The listing builds one solid part. Answer for the finished solid, in the listing's coordinates (mm). Coordinates: 2 decimals unless noted, no trailing zeros. Loops run counter-clockwise (first coordinate to the right, second up) from the corner with the lowest first, then second, coordinate; pieces in that order, holes last. Notation, with made-up numbers: (-18.75, -3) - (16.25, -3) arc R12 ccw to (16.25, 5) - close; hole circle Ø3 at (-31.5, -35). An arc over 180 degrees is marked (long way). Put each result on its own line as item: value.
Autodesk Inventor part; units mm, degrees
ref_plane "YZ Plane" through (0, 0, 0) normal (1, 0, 0) x (0, 1, 0)
ref_plane "XZ Plane" through (0, 0, 0) normal (0, 1, 0) x (-1, 0, 0)
ref_plane "XY Plane" through (0, 0, 0) normal (0, 0, 1) x (1, 0, 0)
sketch "Sketch1" plane through (0, 0, 0) normal (0, 1, 0) x (-1, 0, 0)
  line L0 (25, 100) -> (-25, 100)
  line L1 (-25, 100) -> (-25, -100)
  line L2 (-25, -100) -> (25, -100)
  line L3 (25, -100) -> (25, 100)
  line L4 (25, 100) -> (-25, -100) construction
  line L5 (-25, 100) -> (25, -100) construction
  point P0 (0, 0)
  dimension "d0" = 50
  dimension "d1" = 200
extrude "Extrusion1" add sketch "Sketch1" along normal blind 62
sketch "Sketch2" plane through (-25, 0, 100) normal (0, 0, 1) x (1, 0, 0)
  line L0 (50, 62) -> (0, 62)
  line L1 (50, 62) -> (90, 62)
  line L2 (90, 62) -> (90, 42)
  line L3 (90, 42) -> (53.2289, 0)
  line L4 (53.2289, 0) -> (50, 0)
  line L5 (50, 62) -> (50, 0)
  point P0 (25, 0)
  dimension "d4" = 40
  dimension "d5" = 20
  dimension "d6" = 90
extrude "Extrusion2" add sketch "Sketch2" against normal up to surface (200 mm away)
sketch "Sketch3" plane through (0, 62, 0) normal (0, 1, 0) x (1, 0, 0)
  line L0 (-25, 100) -> (-25, -100)
  line L1 (-25, -100) -> (-25, 100)
  line L2 (-25, 100) -> (-25, 80)
  line L3 (-25, 80) -> (-76.9615, 50)
  line L4 (-25, -100) -> (-25, -80)
  line L5 (-25, -80) -> (-76.9615, -50)
  line L6 (-76.9615, -50) -> (-76.9615, 50)
  circle A0 centre (-76.9615, 0) radius 49.9974
  circle A1 centre (-126.9564, -0.5064) radius 49.9974
  line L7 (-76.9615, -50) -> (-126.45, -50.5013)
  line L8 (-127.4628, 49.4885) -> (-76.9615, 50)
  point P0 (0, 0)
  point P1 (-76.9615, 49.9974)
  point P2 (-77.4679, 49.9949)
  point P3 (-76.9615, -1.0128)
  dimension "d9" = 20
  dimension "d10" = 60
  dimension "d11" = 120
  dimension "d12" = 20
  dimension "d13" = 60
  dimension "d14" = 120
extrude "Extrusion3" add sketch "Sketch3" against normal blind 62
sketch "Sketch4" plane through (0, 62, 0) normal (0, 1, 0) x (1, 0, 0)
  line L0 (-25, -100) -> (28.2289, -100)
  line L1 (-25, 100) -> (-25, 80)
  line L2 (-25, -100) -> (-25, 100)
  line L3 (-25, 100) -> (29.4775, 197.567)
  line L4 (29.4775, 197.567) -> (135.6867, 127.811)
  line L5 (135.6867, 127.811) -> (135.6867, -104.409)
  line L6 (135.6867, -104.409) -> (110.0345, -245.7212)
  line L7 (110.0345, -245.7212) -> (-5.1754, -156.6135)
  line L8 (-5.1754, -156.6135) -> (-25, -100)
  line L9 (-76.9615, -50) -> (-76.9615, 49.9974)
  line L10 (-76.9615, 49.9974) -> (-143.8651, 145.0549)
  line L11 (-143.8651, 145.0549) -> (-248.9816, -0.0013)
  line L12 (-248.9816, -0.0013) -> (-240.1494, -166.1828)
  line L13 (-240.1494, -166.1828) -> (-110.4133, -169.4443)
  line L14 (-110.4133, -169.4443) -> (-76.9615, -50)
  point P0 (0, 0)
extrude "Extrusion4" cut sketch "Sketch4" against normal blind 62 contours L14 L13 L12 L11 L10 L9
extrude "Extrusion5" cut sketch "Sketch4" against normal blind 62 contours L3 L4 L5 L6 L7 L8 L2 L1
properties part number "Piece2" material "Stainless Steel"
1) Straight lines are drawn through the part: L1, parallel to X at y = 10.5, z = 18; L2, parallel to Z at x = -47.5, y = 57.5; L3, parallel to X at y = 8, z = -52. For each, find the intervals that lie inside material, in ascending order. Write a range as [from, to].
Found:
L1: x = [-76.96, -25]
L2: z = [-67.01, 67.01]
L3: x = [-73.5, -25]
2) The part is cut by section B-B (x = -63.5). Give the vertices of the cut face in (y, z), and give its area (3 significant figures).
Found:
outline: (0, -57.77) - (62, -57.77) - (62, 57.77) - (0, 57.77) - close
area: 7,160 mm^2
3) The part is cut by section C-C (z = -53). Give the vertices of the cut face in (x, y).
Found:
outline: (-71.77, 0) - (-25, 0) - (-25, 62) - (-71.77, 62) - close
4) Each of these flat-tipped pins is pushed along its axis until it touches: pin 1 (12 mm diameter, centred on x = -30.5, z = 19, fed in from -Y); pin 2 (4 mm diameter, centred on x = -58, y = 34, fed in from -Z). Where does it stop, or does it pass through?
Found:
pin 1: stops at y = 0
pin 2: stops at z = -62.1
